```python
from build123d import *

# Parameters (mm, degrees)
F0_R           = 9.5
F1_DEPTH       = 1.7
F2_R           = 3.95
F3_DEPTH       = 3.5
F4_SIZE        = 0.5
F5_R           = 0.5
F7_D           = 3.3
F7_CBORE_D     = 6
F7_CBORE_DEPTH = 3


with BuildPart() as f1:
    # F0 (on Front) → F1 (new body)
    with BuildSketch(Plane.XZ):
        Circle(F0_R)
    extrude(amount=F1_DEPTH)

    # F2 (on Front) → F3 (join)
    with BuildSketch(Plane.XZ):
        Circle(F2_R)
    extrude(amount=-F3_DEPTH)

    # F4
    f4_edges = [f1.edges().sort_by_distance(p)[0] for p in [
        (-3.95, 3.5, 0),
        (-9.5, 0, 0),
    ]]
    chamfer(f4_edges, length=F4_SIZE)

    # F5
    f5_edges = [f1.edges().sort_by_distance(p)[0] for p in [
        (-9.5, -1.7, 0),
    ]]
    fillet(f5_edges, radius=F5_R)

    # F7 (through all)
    with Locations(Plane.XZ.offset(1.7)):
        with Locations((0, 0)):
            CounterBoreHole(F7_D / 2, F7_CBORE_D / 2, F7_CBORE_DEPTH)


solid = f1.part
```
Source: CAD feature listing. Evaluate the final solid. Frame: model axes, mm. A direction names the side the tool comes from. Coordinates: 2 decimals unless noted, no trailing zeros. Loops run counter-clockwise (first coordinate to the right, second up) from the corner with the lowest first, then second, coordinate; pieces in that order, holes last. Notation, with made-up numbers: M 43,36 L 84,36 A15 ccw 84,45 Z; hole C 49.5,25 d8. An arc over 180 degrees is marked long. Use a Markdown table: item, result. Add a question column.
Q1. Material intervals for L1, parallel to Z at x = 0, y = 2.2; L2, parallel to Z at x = 0, y = 0.75; L3, parallel to Y at x = 5, z = 3.75, sorted ascending.
Q2. Access query for faces 1 (the flat face through (4, 0, -2)), 2 (the cylindrical face through (4.38, -0.85, -8.43)), 3 (the cylindrical face through (-3, 0, 0)). Directions: +Z, -Z, +X, -X, +Y, -Y. A direction counts if a zero-diameter tool reaches every point of the face in a straight line with its end or side. Return the directions, or none.
Q3. Section query A-A, the plane x = 0. Return loops of the section in (y, z), and give its area (3 significant figures).
Q4. Section query C-C, the plane y = 0.9. Return loops of the section in (x, z).
Q5. Section query B-B, the plane z = 0. Return loops of the section in (x, y).
Q6. Draft query along X for faces 4 (the flat face through (1.3, 1.3, -1.3)), 5 (the cylindrical face through (-3.135, 1.479, -2.404)), 6 (the flat face through (0, -1.7, -4)). Return one class per face: pulls with the +X half, pulls with the -X half, needs draft (parallel to the pull), parting line crosses it, or undercut.
Q7. First-contact query: pin 1 (1 mm diameter, centred on y = -1, z = 5, fed in from +X); pin 2 (2 mm diameter, centred on y = 2, z = 1.5, fed in from +X); pin 3 (3 mm diameter, centred on x = -3, y = 0.5, fed in from +Z); pin 4 (5 mm diameter, centred on x = 1, z = -1, fed in from -Y). Flat tips, straight axial feed; report the tip coordinate or a pass-through.
Result:
| question | item | result |
|---|---|---|
| 1 | L1 | z = -3.95 to -1.65, 1.65 to 3.95 |
| 1 | L2 | z = -3.95 to -3, 3 to 3.95 |
| 1 | L3 | y = -1.7 to 0 |
| 2 | face 1 | +Y |
| 2 | face 2 | +Y, -Y |
| 2 | face 3 | -Y |
| 3 | outline | M -1.7,-9 A0.5 ccw -1.2,-9.5 L -0.5,-9.5 L 0,-9 L 0,-3.95 L 3,-3.95 L 3.5,-3.45 L 3.5,-1.65 L 1.3,-1.65 L 1.3,-3 L -1.7,-3 Z; M -1.7,3 L 1.3,3 L 1.3,1.65 L 3.5,1.65 L 3.5,3.45 L 3,3.95 L 0,3.95 L 0,9 L -0.5,9.5 L -1.2,9.5 A0.5 ccw -1.7,9 Z |
| 3 | area | 34.1 mm2 |
| 4 | outline | C 0,0 d7.9; hole C 0,0 d6 |
| 5 | outline | M -9.5,-1.2 A0.5 ccw -9,-1.7 L -3,-1.7 L -3,1.3 L -1.65,1.3 L -1.65,3.5 L -3.45,3.5 L -3.95,3 L -3.95,0 L -9,0 L -9.5,-0.5 Z; M 1.65,1.3 L 3,1.3 L 3,-1.7 L 9,-1.7 A0.5 ccw 9.5,-1.2 L 9.5,-0.5 L 9,0 L 3.95,0 L 3.95,3 L 3.45,3.5 L 1.65,3.5 Z |
| 6 | face 4 | undercut |
| 6 | face 5 | parting line crosses it |
| 6 | face 6 | needs draft |
| 7 | pin 1 | stops at x = 8.37 |
| 7 | pin 2 | stops at x = 3.92 |
| 7 | pin 3 | stops at z = 9.31 |
| 7 | pin 4 | stops at y = -1.7 |
